from build123d import *

# Parameters (mm, degrees)
SKETCH2_W           = 18.7
SKETCH2_H           = 20
BOSS_EXTRUDE1_DEPTH = 25.4
SKETCH3_W           = 6.35
SKETCH3_H           = 3.175
SKETCH3_H_2         = 4.125
CUT_EXTRUDE1_DEPTH  = 34.653863077
SKETCH5_W           = 3.175
SKETCH5_H           = 25.4
BOSS_EXTRUDE2_DEPTH = 20
SKETCH6_W           = 10
SKETCH6_H           = 10.125
CUT_EXTRUDE2_DEPTH  = 16.825
CUT_EXTRUDE3_REACH  = 34.439
SKETCH7_W           = 3
SKETCH7_H           = 3.5
SKETCH8_W           = 22
SKETCH8_H           = 10.125
CUT_EXTRUDE4_DEPTH  = 19
SKETCH9_W           = 2.175
SKETCH9_H           = 14.925
BOSS_EXTRUDE3_DEPTH = 25.05
SKETCH10_W          = 1.825
SKETCH10_H          = 7.8
CUT_EXTRUDE5_DEPTH  = 4.5
CUT_EXTRUDE6_DEPTH  = 38.694736038
SKETCH15_W          = 0.962350835
SKETCH15_H          = 3.175
CUT_EXTRUDE8_DEPTH  = 10
FILLET1_R           = 3


with BuildPart() as part:
    # Sketch2 → Boss-Extrude1 (new body)
    with BuildSketch(Plane(origin=(0, 0, 0), x_dir=(1, 0, 0), z_dir=(0, 1, 0))):
        Rectangle(SKETCH2_W, SKETCH2_H)
    extrude(amount=BOSS_EXTRUDE1_DEPTH)

    # Sketch3 → Cut-Extrude1 (cut, through all)
    with BuildSketch(Plane(origin=(0, 0, -10), x_dir=(-1, 0, 0), z_dir=(0, 0, -1))):
        with Locations((0, 16.5125)):
            Rectangle(SKETCH3_W, SKETCH3_H)
        with Locations((0, 20.1625)):
            Rectangle(SKETCH3_W, SKETCH3_H_2)
        with Locations((0, 23.8125)):
            Rectangle(SKETCH3_W, SKETCH3_H)
    extrude(amount=-CUT_EXTRUDE1_DEPTH, mode=Mode.SUBTRACT)

    # Sketch5 → Boss-Extrude2 (add)
    with BuildSketch(Plane(origin=(0, 0, -10), x_dir=(-1, 0, 0), z_dir=(0, 0, -1))):
        with Locations((-10.9375, 12.7)):
            Rectangle(SKETCH5_W, SKETCH5_H)
        with Locations((10.9375, 12.7)):
            Rectangle(SKETCH5_W, SKETCH5_H)
    extrude(amount=-BOSS_EXTRUDE2_DEPTH)

    # Sketch6 → Cut-Extrude2 (cut)
    with BuildSketch(Plane(origin=(0, 0, -10), x_dir=(-1, 0, 0), z_dir=(0, 0, -1))):
        Polygon((5, 22.225), (5, 10.125), (5, 0), (9.35, 0), (9.35, 22.225), align=None)
        with Locations((0, 5.0625)):
            Rectangle(SKETCH6_W, SKETCH6_H)
        Polygon((-5, 22.225), (-9.35, 22.225), (-9.35, 0), (-5, 0), (-5, 10.125), align=None)
    extrude(amount=-CUT_EXTRUDE2_DEPTH, mode=Mode.SUBTRACT)

    # Cut-Extrude3: up to this face of the body (flat: up to its plane)
    cut_extrude3_end = Plane(part.part.faces().sort_by_distance((-5, 16.175, -1.5875))[0])
    # Sketch7 → Cut-Extrude3 (cut, up to the picked face)
    with BuildSketch(Plane(origin=(5, 0, 0), x_dir=(0, 0, -1), z_dir=(1, 0, 0)), mode=Mode.PRIVATE) as cut_extrude3_sk1:
        with Locations((-4.825, 19.725)):
            Rectangle(SKETCH7_W, SKETCH7_H)
    cut_extrude3_tool1 = split(extrude(cut_extrude3_sk1.sketch, amount=-CUT_EXTRUDE3_REACH, mode=Mode.PRIVATE), bisect_by=cut_extrude3_end, keep=Keep.BOTH, mode=Mode.PRIVATE)
    add(cut_extrude3_tool1.solids().sort_by(Axis((5, 19.725, 4.825), (-1, 0, 0)))[0], mode=Mode.SUBTRACT)

    # Sketch8 → Cut-Extrude4 (cut)
    with BuildSketch(Plane(origin=(0, 0, -10), x_dir=(-1, 0, 0), z_dir=(0, 0, -1))):
        with Locations((0, 5.0625)):
            Rectangle(SKETCH8_W, SKETCH8_H)
    extrude(amount=-CUT_EXTRUDE4_DEPTH, mode=Mode.SUBTRACT)

    # Sketch9 → Boss-Extrude3 (add)
    with BuildSketch(Plane(origin=(12.525, 0, 0), x_dir=(0, 0, -1), z_dir=(1, 0, 0))):
        with Locations((-11.0875, 7.4625)):
            Rectangle(SKETCH9_W, SKETCH9_H)
    extrude(amount=-BOSS_EXTRUDE3_DEPTH)

    # Sketch10 → Cut-Extrude5 (cut)
    with BuildSketch(Plane(origin=(0, 0, 2.325), x_dir=(-1, 0, 0), z_dir=(0, 0, -1))):
        with Locations((-4.0875, 21.5)):
            Rectangle(SKETCH10_W, SKETCH10_H)
        with Locations((4.0875, 21.5)):
            Rectangle(SKETCH10_W, SKETCH10_H)
    extrude(amount=-CUT_EXTRUDE5_DEPTH, mode=Mode.SUBTRACT)

    # Sketch11 → Cut-Extrude6 (cut, through all)
    with BuildSketch(Plane(origin=(12.525, 0, 0), x_dir=(0, 0, -1), z_dir=(1, 0, 0))):
        Polygon((-10, 14.925), (-6.825, 25.4), (-10, 25.4), align=None)
    extrude(amount=-CUT_EXTRUDE6_DEPTH, mode=Mode.SUBTRACT)

    # Sketch15 → Cut-Extrude8 (cut)
    with BuildSketch(Plane(origin=(-5, 0, 0), x_dir=(0, 0, -1), z_dir=(1, 0, 0))):
        with Locations((-7.306175418, 23.8125)):
            Rectangle(SKETCH15_W, SKETCH15_H)
    extrude(amount=CUT_EXTRUDE8_DEPTH, mode=Mode.SUBTRACT)

    # Fillet1
    # the kernel refuses this fillet: 3 mm, written as the material it takes off along each edge
    with BuildSketch(Plane(origin=(3.175, 32.300803848, 2.325), x_dir=(0, 0, -1), z_dir=(0, -1, 0)), Plane(origin=(-3.175, 17.6, 2.325), x_dir=(0, 0, -1), z_dir=(0, 1, 0))) as fillet1_piece_1:
        with BuildLine():
            CenterArc((2.760321539, 3), FILLET1_R, 203.058244088, 66.941755912)
            Line((0, 1.825), (-0.055206431, 1.8015))
            ThreePointArc((-0.055206431, 1.8015), (-0.06, 0.9125), (-0.06, 0))
            Line((-0.06, 0), (0, -0.06))
            Line((0, -0.06), (2.760321539, -0.06))
            Line((2.760321539, -0.06), (2.760321539, 0))
        make_face()
    extrude(amount=14.700803848, mode=Mode.SUBTRACT)


solid = part.part
The model under review builds one solid part; all positions refer to its coordinate system, in mm. A direction names the side the tool comes from. Round coordinates to 2 decimals unless told otherwise and drop trailing zeros. Order: outer loops, then holes, each group sorted by start corner. A loop starts at its lowest first (then second) coordinate and runs counter-clockwise, first axis right, second up. Notation, with made-up numbers: (47.25, -15) -> (72.25, -15) arc R22 cw to (72.25, -1) -> close; hole circle Ø9 at (67, 47). An arc over 180 degrees is marked (long way). Use CSV: the item, a comma, the result in double quotes. Start each with the question number.
(1) Tool access review of faces 1 (the face through (-5, 16, -2)), 2 (the face through (4, 22.225, 7)), 3 (the face through (-7.785, 20.089, 8.435)), 4 (the face through (-3.175, 19, -2)): name each direction out of +Z, -Z, +X, -X, +Y, -Y from which nothing blocks a thin tool from reaching the whole face with its end or side.
(2) Consider section C-C on x = 5.75. Write out the cut boundary in (y, z) (3 decimals), and give its area (3 significant figures).
(3) Wall thickness on probe 1 along X at (y, z) = (16.25, -7.5) (3 decimals); probe 2 along X at (y, z) = (11.75, -3.25) (3 decimals); probe 3 along X at (y, z) = (3.5, -1.5) (3 decimals): over which ranges is each line inside the solid? List them lowest first. Write a range as from..to.
(4) Mouldability with a two-part tool opening along X and no side actions: class faces 5 (the face through (0, 5, 9)), 6 (the face through (-12.525, 13, 1)), 7 (the face through (7, 16, 6.825)), 8 (the face through (-0.9, 14.6, -10)) as pulls with the +X half, pulls with the -X half, needs draft (parallel to the pull), parting line crosses it, or undercut.
(5) Consider section D-D on y = 15.5. Write out the cut boundary in (x, z) (3 decimals), and give its area (3 significant figures).
(6) Insertion check: pin 1 (1.9 mm diameter, centred on x = 7.5, y = 19, fed in from -Z) (3 decimals); pin 2 (1.5 mm diameter, centred on x = 4, z = 3, fed in from +Y); pin 3 (1.5 mm diameter, centred on x = -5.5, z = 4, fed in from -Y) (3 decimals). Each pin has a flat end and moves straight along its axis. Give the tip position at first contact, or say it passes through.
(7) Consider section B-B on y = 12.25. Write out the cut boundary in (x, z) (3 decimals).
(8) Consider section A-A on z = 6. Write out the cut boundary in (x, y) (3 decimals), and give its area (3 significant figures).
Responses:
1,face 1,"-Z, -Y"
1,face 2,"+Z, +Y"
1,face 3,"+Z, +X, -X, +Y"
1,face 4,"+Z, -Z, +Y"
2,outline,"(0, 9) -> (10.125, 9) -> (10.125, 6.825) -> (22.225, 6.825) -> (22.225, -10) -> (25.4, -10) -> (25.4, 6.825) -> (14.925, 10) -> (14.925, 12.175) -> (0, 12.175) -> close"
2,area,"128 mm²"
3,probe 1,"-12.525..-9.35, -5..-3.175, 3.175..5, 9.35..12.525"
3,probe 2,"-12.525..-9.35, -5..5, 9.35..12.525"
3,probe 3,"-12.525..-11, 11..12.525"
4,face 5,"undercut"
4,face 6,"pulls with the -X half"
4,face 7,"undercut"
4,face 8,"needs draft"
5,outline,"(-12.525, -10) -> (-9.35, -10) -> (-9.35, 6.825) -> (-5, 6.825) -> (-5, -10) -> (-3.175, -10) -> (-3.175, 9.826) -> (-12.525, 9.826) -> close; (3.175, -10) -> (5, -10) -> (5, 6.825) -> (9.35, 6.825) -> (9.35, -10) -> (12.525, -10) -> (12.525, 9.826) -> (3.175, 9.826) -> close"
5,area,"224 mm²"
6,pin 1,"z = 6.825"
6,pin 2,"y = 17.6"
6,pin 3,"y = 10.125"
7,outline,"(-12.525, -10) -> (-9.35, -10) -> (-9.35, 6.825) -> (-5, 6.825) -> (-5, -10) -> (5, -10) -> (5, 6.825) -> (9.35, 6.825) -> (9.35, -10) -> (12.525, -10) -> (12.525, 12.175) -> (-12.525, 12.175) -> close"
8,outline,"(-12.525, 0) -> (-11, 0) -> (-11, 10.125) -> (-9.35, 10.125) -> (-9.35, 22.225) -> (-5, 22.225) -> (-5, 25.4) -> (-12.525, 25.4) -> close; (-5, 10.125) -> (5, 10.125) -> (5, 17.6) -> (3.175, 17.6) -> (3.175, 14.925) -> (-3.175, 14.925) -> (-3.175, 17.6) -> (-5, 17.6) -> close; (5, 22.225) -> (9.35, 22.225) -> (9.35, 10.125) -> (11, 10.125) -> (11, 0) -> (12.525, 0) -> (12.525, 25.4) -> (5, 25.4) -> close"
8,area,"213 mm²"
